CAD build for the part. Positions are in the model's coordinates, mm. A direction names the side the tool comes from. Round coordinates to 2 decimals unless told otherwise and drop trailing zeros. Order: outer loops, then holes, each group sorted by start corner. A loop starts at its lowest first (then second) coordinate and runs counter-clockwise, first axis right, second up. Notation, with made-up numbers: M 44,-19.5 L 83,-19.5 A8 ccw 83,-7.5 Z; hole C 34.25,72.5 d9. An arc over 180 degrees is marked long. Answer as a JSON object with one key per item and string values.
```python
from build123d import *

# Parameters (mm, degrees)
F0_W     = 1460.5
F0_H     = 755.65
F0_H_2   = 6.35
F1_DEPTH = 38.1
F2_DEPTH = 723.9
F3_DEPTH = 635
F4_R     = 19.04999
F5_R     = 5.08


# Not quite as in the source:
# - a fillet or chamfer is up to 0.001 mm smaller than in the source, because OpenCascade refuses the exact size


with BuildPart() as f1:
    # F0 (on Top) → F1 (new body)
    with BuildSketch(Plane.XY):
        with Locations((762, 377.825)):
            Rectangle(F0_W, F0_H)
        Polygon((0, 762), (0, 0), (31.75, 0), (31.75, 755.65), (31.75, 762), align=None)
        with Locations((762, 758.825)):
            Rectangle(F0_W, F0_H_2)
        Polygon((1492.25, 755.65), (1492.25, 0), (1524, 0), (1524, 762), (1492.25, 762), align=None)
    extrude(amount=F1_DEPTH)

    # F0 (on Top) → F2 (join)
    with BuildSketch(Plane.XY):
        Polygon((0, 762), (0, 0), (31.75, 0), (31.75, 755.65), (31.75, 762), align=None)
        Polygon((1492.25, 755.65), (1492.25, 0), (1524, 0), (1524, 762), (1492.25, 762), align=None)
    extrude(amount=-F2_DEPTH)

    # F0 (on Top) → F3 (join)
    with BuildSketch(Plane.XY):
        with Locations((762, 758.825)):
            Rectangle(F0_W, F0_H_2)
    extrude(amount=-F3_DEPTH)

    # F4 (radius 19.05 in the source; OpenCascade refuses exactly that, so slightly less here)
    f4_edges = [f1.edges().sort_by_distance(p)[0] for p in [
        (762, 0, 38.1),
        (762, 0, 0),
    ]]
    fillet(f4_edges, radius=F4_R)

    # F5
    f5_edges = [f1.edges().sort_by_distance(p)[0] for p in [
        (1524, 0, -352.424995),
        (762, 0, 19.05001),
        (1508.125, 0, -723.9),
        (0, 0, -352.424995),
        (1492.25, 0, -361.95),
        (15.875, 0, -723.9),
        (1492.25, 0, 9.524995),
        (31.75, 0, -361.95),
        (762, 0, 19.04999),
        (31.75, 0, 9.524995),
    ]]
    fillet(f5_edges, radius=F5_R)


solid = f1.part
```
Item 1: Wall check: line 1 along X through (y, z) = (588, -659); line 2 along Z through (x, y) = (1366.5, 337.5); line 3 along Y through (x, z) = (1296.5, -147.5). Give the ranges that are in metal, low to high. Write a range as [from, to].
Worked answers:
{"line 1": "x = [0, 31.75], [1492.25, 1524]", "line 2": "z = [0, 38.1]", "line 3": "y = [755.65, 762]"}
Item 2: Saw through at B-B on z = -669. List the corners of the cut face in (x, y).
Worked answers:
{"outline": "M 0,5.08 A5.08 ccw 5.08,0 L 26.67,0 A5.08 ccw 31.75,5.08 L 31.75,762 L 0,762 Z; M 1492.25,5.08 A5.08 ccw 1497.33,0 L 1518.92,0 A5.08 ccw 1524,5.08 L 1524,762 L 1492.25,762 Z"}
Item 3: Saw through at D-D on z = -102.5. List the corners of the cut face in (x, y).
Worked answers:
{"outline": "M 0,5.08 A5.08 ccw 5.08,0 L 26.67,0 A5.08 ccw 31.75,5.08 L 31.75,755.65 L 1492.25,755.65 L 1492.25,5.08 A5.08 ccw 1497.33,0 L 1518.92,0 A5.08 ccw 1524,5.08 L 1524,762 L 0,762 Z"}
Item 4: Saw through at A-A on y = 429. List the corners of the cut face in (x, z).
Worked answers:
{"outline": "M 0,-723.9 L 31.75,-723.9 L 31.75,0 L 1492.25,0 L 1492.25,-723.9 L 1524,-723.9 L 1524,33.02 A5.08 ccw 1518.92,38.1 L 5.08,38.1 A5.08 ccw 0,33.02 Z"}
Item 5: 3-axis set-ups, long thin cutter, end or side, ignore diameter. For faces 1 (the flat face through (752, 393, 0)), 2 (the flat face through (1524, 378, -351)): which of +Z, -Z, +X, -X, +Y, -Y reach the whole face in a straight line?
Worked answers:
{"face 1": "-Z, -Y", "face 2": "+Z, -Z, +X, +Y, -Y"}
Item 6: Drop flat-ended pins along their axis: pin 1 Ø10 at (x, z) = (934.5, -164) entering from -Y; pin 2 Ø7 at (x, y) = (868, 759) entering from -Z. Give the stop position or say it passes through.
Worked answers:
{"pin 1": "stops at y = 755.65", "pin 2": "stops at z = -635"}
Item 7: Two-plate mould, pull along X, no slides. Class faces 3 (the flat face through (1492.25, 389, -354)), 4 (the flat face through (0, 389, -340)), 5 (the flat face through (1508, 389, -723.9)), 6 (the flat face through (31.75, 378, -354)): released by +X, released by -X, zero draft, split by the parting line, or undercut.
Worked answers:
{"face 3": "undercut", "face 4": "released by -X", "face 5": "zero draft", "face 6": "undercut"}
